Geometry: final body of the model. Coordinates: model frame, mm. Face numbers are marked on the shaded views. A direction names the side the tool comes from. Round coordinates to 2 decimals unless told otherwise and drop trailing zeros. Loops run counter-clockwise (first coordinate to the right, second up) from the corner with the lowest first, then second, coordinate; pieces in that order, holes last. Notation, with made-up numbers: M -38,44 L -30,44 A20 cw -30,71 Z; hole C 60,-1 d3. An arc over 180 degrees is marked long. Answer as a JSON object with one key per item and string values.
```python
from build123d import *

# Parameters (mm, degrees)
F0_R     = 1.7272
F0_R_2   = 1.0407250193
F1_DEPTH = 4.7625
F3_DEPTH = 7.9375
F4_R     = 1.7272
F5_DEPTH = 7.9375


with BuildPart() as f1:
    # F0 (on Top) → F1 (new body)
    with BuildSketch(Plane.XY):
        with BuildLine():
            Line((-2.0541653616, 1.330521752), (0, 0))
            Line((0, 0), (-79.738154648, 0))
            Line((-79.738154648, 0), (-75.2879145345, 4.4502401135))
            ThreePointArc((-75.2879145345, 4.4502401135), (-75.2879145345, 10.0629001892), (-80.9005746101, 10.0629001892))
            Line((-80.9005746101, 10.0629001892), (-92.1258947615, -1.1624199622))
            ThreePointArc((-92.1258947615, -1.1624199622), (-92.9862116183, -5.4875248722), (-89.3195647236, -7.9375))
            Line((-89.3195647236, -7.9375), (13.4275761574, -7.9375))
            ThreePointArc((13.4275761574, -7.9375), (17.2335612406, -5.093674046), (15.5851543061, -0.6377091574))
            Line((15.5851543061, -0.6377091574), (2.2609909357, 7.9926034372))
            ThreePointArc((2.2609909357, 7.9926034372), (-3.2276280555, 6.8191407432), (-2.0541653616, 1.330521752))
        make_face()
        with Locations((-89.3195647236, -3.96875)):
            Circle(F0_R, mode=Mode.SUBTRACT)
        with Locations((13.4275761574, -3.96875)):
            Circle(F0_R, mode=Mode.SUBTRACT)
        with Locations((6.7654944722, 0.3464062973)):
            Circle(F0_R_2, mode=Mode.SUBTRACT)
        with Locations((-78.0942445723, 7.2565701513)):
            Circle(F0_R, mode=Mode.SUBTRACT)
        with Locations((0.1034127871, 4.6615625946)):
            Circle(F0_R, mode=Mode.SUBTRACT)
    extrude(amount=F1_DEPTH)

    # F2 (on face) → F3 (join, through all)
    with BuildSketch(Plane.XZ.offset(7.9375)):
        with BuildLine():
            Line((-75.0487659739, 4.7625), (-68.3135738831, 4.7625))
            Line((-68.3135738831, 4.7625), (-61.5783817923, 4.7625))
            Line((-61.5783817923, 4.7625), (-64.9459778377, 8.1300960454))
            ThreePointArc((-64.9459778377, 8.1300960454), (-68.3135738831, 9.525), (-71.6811699285, 8.1300960454))
            Line((-71.6811699285, 8.1300960454), (-75.0487659739, 4.7625))
        make_face()
        with BuildLine():
            Line((-14.3136067739, 4.7625), (-7.5784146831, 4.7625))
            Line((-7.5784146831, 4.7625), (-0.8432225923, 4.7625))
            Line((-0.8432225923, 4.7625), (-4.2108186377, 8.1300960454))
            ThreePointArc((-4.2108186377, 8.1300960454), (-7.5784146831, 9.525), (-10.9460107285, 8.1300960454))
            Line((-10.9460107285, 8.1300960454), (-14.3136067739, 4.7625))
        make_face()
    extrude(amount=-F3_DEPTH)

    # F4 (on face) → F5 (cut, through all)
    with BuildSketch(Plane.XZ.offset(7.9375)):
        with Locations((-68.3135738831, 4.7625)):
            Circle(F4_R)
        with Locations((-7.5784146831, 4.7625)):
            Circle(F4_R)
    extrude(amount=-F5_DEPTH, mode=Mode.SUBTRACT)


solid = f1.part
```
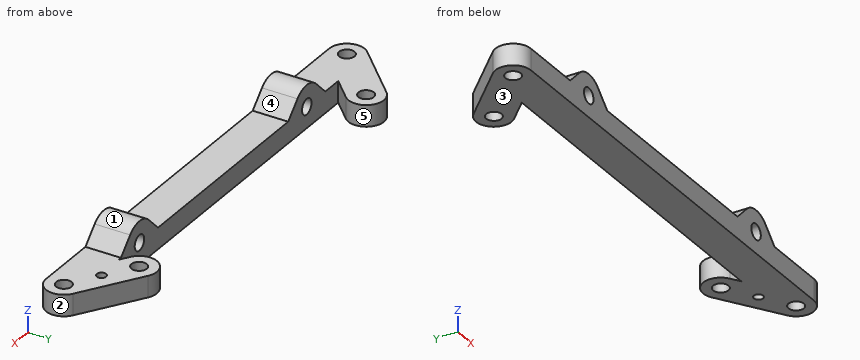
1) Cut plane A-A on x = -29. Return the cut outline in (y, z).
Geometry results:
{"outline": "M -7.94,0 L 0,0 L 0,4.76 L -7.94,4.76 Z"}
2) First-contact query: pin 1 (5.5 mm diameter, centred on x = -78.09, y = 7.26, fed in from +Z); pin 2 (3 mm diameter, centred on x = 0.1, y = 4.66, fed in from +Z) (3 decimals); pin 3 (4 mm diameter, centred on x = -7.58, z = 4.76, fed in from +Y); pin 4 (3 mm diameter, centred on y = -1, z = 8, fed in from +X). Flat tips, straight axial feed; report the tip coordinate or a pass-through.
Geometry results:
{"pin 1": "z = 4.76", "pin 2": "through", "pin 3": "y = 0", "pin 4": "x = -2.58"}
3) Pull-direction query (X, two-part tool) for the marked faces 1, 2 and 3; classes: +X half, -X half, draft (parallel to the pull), parting line (faces both ways), or undercut.
Geometry results:
{"face 1": "undercut", "face 2": "+X half", "face 3": "draft"}
4) Cut plane B-B on x = -86. Return the cut outline in (y, z).
Geometry results:
{"outline": "M -7.94,0 L 4.96,0 L 4.96,4.76 L -7.94,4.76 Z"}
5) Set-up query: the marked faces 4 and 5. Return all of +Z, -Z, +X, -X, +Y, -Y with unobstructed straight access to the full face (end or side cutting, diameter ignored); none if empty.
Geometry results:
{"face 4": "+Z, +Y, -Y", "face 5": "+Z, -Z"}
6) Line query: probe 1 along X at (y, z) = (-2, 6); probe 2 along X at (y, z) = (5, 2.25); probe 3 along Y at (x, z) = (-79.5, 1.25). Output: solid intervals per line, ascending.
Geometry results:
{"probe 1": "-73.81 to -69.52, -67.11 to -62.82, -13.08 to -8.78, -6.37 to -2.08", "probe 2": "-85.96 to -74.83, -3.85 to -1.59, 1.8 to 6.88", "probe 3": "-7.94 to 0, 0.24 to 6.25, 8.26 to 10.97"}
